Source: CAD feature listing. Evaluate the final solid. Frame: model axes, mm. A direction names the side the tool comes from. Give positions to 0.01 mm unless a question says otherwise; leave off trailing zeros. Loops run counter-clockwise (first coordinate to the right, second up) from the corner with the lowest first, then second, coordinate; pieces in that order, holes last.
from build123d import *

# Parameters (mm, degrees)
SKETCH_1_W          = 28
SKETCH_1_H          = 28
EXTRUDE_1_DEPTH     = 3.5
SKETCH_2_W          = 4
SKETCH_2_H          = 28
EXTRUDE_2_DEPTH     = 25
SKETCH_3_R          = 9
CUT_EXTRUDE_1_DEPTH = 50
SKETCH_4_R          = 1.55
CUT_EXTRUDE_2_DEPTH = 50


with BuildPart() as part:
    # 草图1 → 凸台-拉伸1 (new body)
    with BuildSketch(Plane(origin=(0, 0, 0), x_dir=(1, 0, 0), z_dir=(0, 1, 0))):
        with Locations((14, -14)):
            Rectangle(SKETCH_1_W, SKETCH_1_H)
    extrude(amount=EXTRUDE_1_DEPTH)

    # 草图2 → 凸台-拉伸2 (add)
    with BuildSketch(Plane(origin=(0, 3.5, 0), x_dir=(1, 0, 0), z_dir=(0, 1, 0))):
        with Locations((2, -14)):
            Rectangle(SKETCH_2_W, SKETCH_2_H)
        with Locations((26, -14)):
            Rectangle(SKETCH_2_W, SKETCH_2_H)
    extrude(amount=EXTRUDE_2_DEPTH)

    # 草图3 → 切除-拉伸1 (cut)
    with BuildSketch(Plane.ZY):
        with Locations((15, 16.5)):
            Circle(SKETCH_3_R)
    extrude(amount=-CUT_EXTRUDE_1_DEPTH, mode=Mode.SUBTRACT)

    # 草图4 → 切除-拉伸2 (cut)
    with BuildSketch(Plane(origin=(0, 3.5, 0), x_dir=(1, 0, 0), z_dir=(0, 1, 0))):
        with Locations(Location((12, -19, 0), (0, 0, 270))):
            Circle(SKETCH_4_R)
        with Locations(Location((12, -9, 0), (0, 0, 270))):
            Circle(SKETCH_4_R)
    extrude(amount=-CUT_EXTRUDE_2_DEPTH, mode=Mode.SUBTRACT)


solid = part.part
1) Contact query for flat-ended pins moving along their axis: P1, Ø3, axis at x = 7, y = 5.5, coming from the -Z side; P2, Ø1, axis at x = 5, z = 24.5, coming from the +Y side. Output: stop coordinate, or through.
Checks:
P1: passes through
P2: stops at y = 3.5
2) Cut plane D-D (x = 2). Return loops of the section in (y, z), and give its area (3 significant figures).
Checks:
outline: (0, 0) - (28.5, 0) - (28.5, 28) - (0, 28) - close; hole circle Ø18 at (16.5, 15)
area: 544 mm2
3) Pull-direction query (Z, two-part tool) for faces 3 (the flat face through (0, 8, 11)), 4 (the cylindrical face through (11.406, 1.774, 20.432)), 5 (the flat face through (3.6, 11, 28)); classes: released by +Z, released by -Z, zero draft, split by the parting line, or undercut.
Checks:
face 3: zero draft
face 4: undercut
face 5: released by +Z
4) Reachability of faces 1 (the flat face through (3.6, 11, 0)), 2 (the flat face through (4, 10, 8)) from +Z, -Z, +X, -X, +Y, -Y: full face, straight path, thin tool, end or side. Return the list, or none.
Checks:
face 1: -Z, +X, -X, +Y, -Y
face 2: +Z, -Z, +Y
5) Cut plane C-C (x = 12). Return loops of the section in (y, z), and give its area (3 significant figures).
Checks:
outline: (0, 0) - (3.5, 0) - (3.5, 7.45) - (0, 7.45) - close; (0, 10.55) - (3.5, 10.55) - (3.5, 17.45) - (0, 17.45) - close; (0, 20.55) - (3.5, 20.55) - (3.5, 28) - (0, 28) - close
area: 76.3 mm2
6) Cut plane A-A (y = 16.5). Return loops of the section in (x, z).
Checks:
outline: (0, 0) - (4, 0) - (4, 6) - (0, 6) - close; (0, 24) - (4, 24) - (4, 28) - (0, 28) - close; (24, 0) - (28, 0) - (28, 6) - (24, 6) - close; (24, 24) - (28, 24) - (28, 28) - (24, 28) - close
7) Cut plane B-B (z = 19). Return loops of the section in (x, y), and give its area (3 significant figures).
Checks:
outline: (0, 0) - (10.45, 0) - (10.45, 3.5) - (4, 3.5) - (4, 8.44) - (0, 8.44) - close; (0, 24.56) - (4, 24.56) - (4, 28.5) - (0, 28.5) - close; (13.55, 0) - (28, 0) - (28, 8.44) - (24, 8.44) - (24, 3.5) - (13.55, 3.5) - close; (24, 24.56) - (28, 24.56) - (28, 28.5) - (24, 28.5) - close
area: 158 mm2
8) Ray query, probe 1 along X at (y, z) = (2.15, 19); probe 2 along X at (y, z) = (25.5, 12.5); probe 3 along Y at (x, z) = (7, 14.25). Return the intervals inside material, ascending.
Checks:
probe 1: x = 0 to 10.45, 13.55 to 28
probe 2: x = 0 to 4, 24 to 28
probe 3: y = 0 to 3.5
